Autodesk Inventor part; units mm, degrees
ref_plane "YZ Plane" through (0, 0, 0) normal (1, 0, 0) x (0, 1, 0)
ref_plane "XZ Plane" through (0, 0, 0) normal (0, 1, 0) x (-1, 0, 0)
ref_plane "XY Plane" through (0, 0, 0) normal (0, 0, 1) x (1, 0, 0)
sketch "Boceto1" plane through (0, 0, 0) normal (0, 0, 1) x (1, 0, 0)
  line L0 (0, 0) -> (4, 0)
  line L1 (4, 0) -> (4, 12.5)
  line L2 (4, 12.5) -> (0, 12.5)
  line L3 (0, 12.5) -> (0, 0)
  line L4 (0, 12.5) -> (5, 12.5)
  line L5 (5, 12.5) -> (5, 14.5)
  line L6 (5, 14.5) -> (0, 14.5)
  line L7 (0, 14.5) -> (0, 12.5)
  point P0 (4, 12.5)
  dimension "d0" = 4
  dimension "d1" = 12.5
  dimension "d2" = 5
  dimension "d3" = 2
revolve "Revolución1" add sketch "Boceto1" angle 360 about axis through (0, 12.5, 0) along (0, -1, 0)
thread "Rosca1"
sketch "Boceto2" plane through (0, 14.5, 0) normal (0, 1, 0) x (1, 0, 0)
  line L0 (-0.5, -5) -> (0.5, -5)
  line L1 (0.5, -5) -> (0.5, 5)
  line L2 (0.5, 5) -> (-0.5, 5)
  line L3 (-0.5, 5) -> (-0.5, -5)
  line L4 (5, -0.5) -> (-5, -0.5)
  line L5 (-5, -0.5) -> (-5, 0.5)
  line L6 (-5, 0.5) -> (5, 0.5)
  line L7 (5, 0.5) -> (5, -0.5)
  point P0 (0, 0)
  point P1 (0.5, 0.5)
  point P2 (0.5, -0.5)
  point P3 (-0.5, -0.5)
  point P4 (-0.5, 0.5)
  dimension "d7" = 1
  dimension "d8" = 1
  dimension "d9" = 10
  dimension "d10" = 10
  dimension "d11" = 0.5
  dimension "d12" = 0.5
  dimension "d13" = 5
  dimension "d14" = 5
extrude "Extrusión1" cut sketch "Boceto2" against normal blind 1
fillet "Empalme1" radius 1 1 edges at (3.5355, 14.5, -3.5355)
fillet "Empalme2" radius 1 3 edges at (-3.5355, 14.5, -3.5355) (-3.5355, 14.5, 3.5355) (3.5355, 14.5, 3.5355)
equation "\"d8\" = d7"
equation "\"d10\" = d9"
properties part number "Tornillo" material "Acero inoxidable"
For this review, take the finished solid that the model builds, in its own axes (mm). A direction names the side the tool comes from. Coordinates: 2 decimals unless noted, no trailing zeros. Loops run counter-clockwise (first coordinate to the right, second up) from the corner with the lowest first, then second, coordinate; pieces in that order, holes last. Notation, with made-up numbers: (24.25, 29.25) -> (48.25, 29.25) arc R12 ccw to (48.25, 50.25) -> close; hole circle Ø4 at (9.5, 11). An arc over 180 degrees is marked (long way). Return JSON: item names as keys, results as strings. Group by question number.
(1) Consider section C-C, the plane y = 12.75. Give the boundary of the cut face in (x, z), plus the area to 3 significant figures.
(2) Consider section B-B, the plane x = 0. Give the boundary of the cut face in (y, z).
(3) Mouldability with a two-part tool opening along Z and no side actions: class faces 1 (the flat face through (0.5, 14, -3)), 2 (the cylindrical face through (-0.867, 6.338, 3.905)), 3 (the flat face through (-3, 14, 0.5)) as pulls with the +Z half, pulls with the -Z half, needs draft (parallel to the pull), parting line crosses it, or undercut.
(4) For pin 1 Ø0.5 at (y, z) = (14, 2) entering from +X; pin 2 Ø5 at (y, z) = (5, 4) entering from -X; pin 3 Ø0.8 at (y, z) = (14, -2) entering from +X; pin 4 Ø1.5 at (x, z) = (-2, 0) entering from +Y, all flat-tipped, find the tip position at first contact; note any pin that passes through.
(5) Tool access review of faces 4 (the flat face through (3, 14, 0.5)), 5 (the flat face through (-0.5, 14, 3)), 6 (the flat face through (-2, 14.5, -2)): name each direction out of +Z, -Z, +X, -X, +Y, -Y from which nothing blocks a thin tool from reaching the whole face with its end or side.
(6) Consider section D-D, the plane y = 4.5. Give the boundary of the cut face in (x, z).
(7) To check wall thickness, follow L1, parallel to X at y = 8.5, z = -0.5; L2, parallel to Z at x = -1.5, y = 13.75. State the ranges of each line that lie inside material, in increasing order.
(8) Consider section A-A, the plane z = 0. Give the boundary of the cut face in (x, y), plus the area to 3 significant figures.
Results below:
{
 "1": {"outline": "circle Ø10 at (0, 0)", "area": "78.5 mm2"},
 "2": {"outline": "(0, -4) -> (12.5, -4) -> (12.5, -5) -> (13.5, -5) -> (13.5, 5) -> (12.5, 5) -> (12.5, 4) -> (0, 4) -> close"},
 "3": {"face 1": "needs draft", "face 2": "parting line crosses it", "face 3": "undercut"},
 "4": {"pin 1": "stops at x = 4.6", "pin 2": "stops at x = -3.71", "pin 3": "stops at x = 4.67", "pin 4": "stops at y = 14.5"},
 "5": {"face 4": "+X, -X, +Y", "face 5": "+Z, -Z, +Y", "face 6": "+Z, -Z, +X, -X, +Y"},
 "6": {"outline": "circle Ø8 at (0, 0)"},
 "7": {"L1": "x = -3.97 to 3.97", "L2": "z = -4.74 to -0.5, 0.5 to 4.74"},
 "8": {"outline": "(-5, 12.5) -> (-4, 12.5) -> (-4, 0) -> (4, 0) -> (4, 12.5) -> (5, 12.5) -> (5, 13.5) -> (-5, 13.5) -> close", "area": "110 mm2"}
}
